Read the model definition and answer for the solid it produces. Units are mm, in the model's axes. Coordinates: 2 decimals unless noted, no trailing zeros. Write each loop counter-clockwise with the first axis right and the second up, starting at its lowest first coordinate (ties: lowest second). Pieces come first, ordered by that corner, then holes.
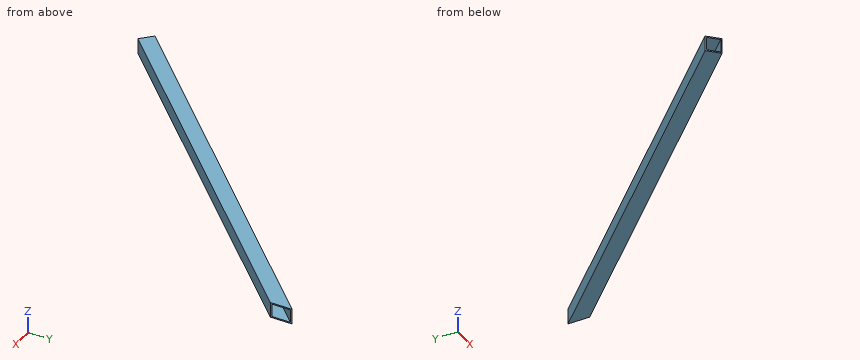
Autodesk Inventor part; units mm, degrees
ref_plane "YZ Plane" through (0, 0, 0) normal (1, 0, 0) x (0, 1, 0)
ref_plane "XZ Plane" through (0, 0, 0) normal (0, 1, 0) x (-1, 0, 0)
ref_plane "XY Plane" through (0, 0, 0) normal (0, 0, 1) x (1, 0, 0)
sketch "Sketch2" plane through (0, 0, 0) normal (0, 0, 1) x (1, 0, 0)
  line L0 (0, 0) -> (377.5, 0) construction
  line L1 (377.5, 0) -> (377.5, 377.5) construction
  line L2 (0, 0) -> (377.5, 377.5) construction
  line L3 (-6.7175, 6.7175) -> (6.7175, -6.7175)
  line L4 (377.5, 390.935) -> (377.5, 364.065)
  line L5 (-6.7175, 6.7175) -> (377.5, 390.935)
  line L6 (6.7175, -6.7175) -> (377.5, 364.065)
  dimension "d4" = 377.5
  dimension "d5" = 377.5
  dimension "d6" = 19
  dimension "d7" = 90
  dimension "d13" = 45
extrude "Extrusion1" add sketch "Sketch2" along normal blind 19
sketch "Sketch3" plane through (6.7175, -6.7175, 19) normal (-0.7071, -0.7071, 0) x (-0.7071, 0.7071, 0)
  line L0 (19, 19) -> (0, 19)
  line L1 (0, 19) -> (0, 0)
  line L2 (19, 0) -> (0, 0)
  line L3 (19, 19) -> (19, 0)
  line L4 (17.5, 1.5) -> (1.5, 1.5)
  line L5 (1.5, 1.5) -> (1.5, 17.5)
  line L6 (1.5, 17.5) -> (17.5, 17.5)
  line L7 (17.5, 17.5) -> (17.5, 1.5)
  point P0 (9.5, 19)
  dimension "d14" = 1.5
extrude "Extrusion2" cut sketch "Sketch3" against normal through all contours L4 L5 L6 L7
properties part number "C004" material "Aluminum 6061"
Item 1: Given pin 1 (2 mm diameter, centred on y = 41, z = 14.5, fed in from +X) (3 decimals); pin 2 (2 mm diameter, centred on x = 139, z = 15, fed in from -Y) (3 decimals); pin 3 (10 mm diameter, centred on y = 187, z = 4.5, fed in from +X) (3 decimals), each flat-ended and moving along its own axis, determine where each tip first touches the part or whether it passes through.
Item 2: The part is cut by section C-C (x = 254). Give the vertices of the cut face in (y, z) (3 decimals).
Item 3: The part is cut by section B-B (y = 90.5). Give the vertices of the cut face in (x, z) (3 decimals), and give its area (3 significant figures).
Item 4: The part is cut by section A-A (z = 12.5). Give the vertices of the cut face in (x, y) (1 decimal), and give its area (3 significant figures).
Item 5: Find the intervals of material crossed by probe 1 along Z at (x, y) = (266, 274.5); probe 2 along Y at (x, z) = (198, 5.75) (3 decimals); probe 3 along X at (y, z) = (255.5, 7) (3 decimals), in increasing order.
Answer:
1. pin 1: stops at x = 55.435
1. pin 2: stops at y = 124.565
1. pin 3: stops at x = 205.435
2. outline: (240.565, 0) - (267.435, 0) - (267.435, 19) - (240.565, 19) - close; hole (242.686, 1.5) - (265.314, 1.5) - (265.314, 17.5) - (242.686, 17.5) - close
3. outline: (77.065, 0) - (103.935, 0) - (103.935, 19) - (77.065, 19) - close; hole (79.186, 1.5) - (101.814, 1.5) - (101.814, 17.5) - (79.186, 17.5) - close
3. area: 148 mm2
4. outline: (-6.7, 6.7) - (-5.7, 5.7) - (377.5, 388.8) - (377.5, 390.9) - close; (5.7, -5.7) - (6.7, -6.7) - (377.5, 364.1) - (377.5, 366.2) - close
4. area: 1,600 mm2
5. probe 1: z = 0 to 1.5, 17.5 to 19
5. probe 2: y = 184.565 to 186.686, 209.314 to 211.435
5. probe 3: x = 242.065 to 244.186, 266.814 to 268.935
